Autodesk Inventor part; units mm, degrees
ref_plane "YZ Plane" through (0, 0, 0) normal (1, 0, 0) x (0, 1, 0)
ref_plane "XZ Plane" through (0, 0, 0) normal (0, 1, 0) x (-1, 0, 0)
ref_plane "XY Plane" through (0, 0, 0) normal (0, 0, 1) x (1, 0, 0)
sketch "Sketch1" plane through (0, 0, 0) normal (0, 0, 1) x (1, 0, 0)
  line L0 (-4, 26) -> (-4, -4)
  line L1 (-4, -4) -> (16, -4)
  line L2 (16, -4) -> (16, 0)
  line L3 (16, 0) -> (0, 0)
  line L4 (0, 0) -> (0, 26)
  line L5 (0, 26) -> (-4, 26)
  point P0 (0, 0)
  dimension "d0" = 30
  dimension "d1" = 20
  dimension "d2" = 4
  dimension "d3" = 4
extrude "Extrusion1" add sketch "Sketch1" along normal mid plane 120
sketch "Sketch2" plane through (0, 0, 0) normal (0, 0, 1) x (1, 0, 0)
  line L0 (0, 0) -> (0, 26)
  line L1 (16, -4) -> (16, 0)
  line L2 (0, 26) -> (16, 0)
  line L3 (16, 0) -> (0, 0)
extrude "Extrusion2" add sketch "Sketch2" along normal mid plane 4
fillet "Fillet1" radius 2 8 edges at (0, 0, 31) (0, 0, -31) (0, 13, 2) (8, 0, 2) (0, 13, -2) (8, 0, -2) (-2, 26, 60) (-2, 26, -60)
sketch "Sketch3" plane through (0, 2, 4) normal (1, 0, 0) x (0, 0, -1)
  line L0 (64, -6) -> (-56, -6)
  line L1 (8, 24) -> (0, 24)
  point P0 (4, -2)
  point P1 (-38.5, 12.28)
  point P2 (4, 24)
  dimension "d19" = 18.28
  dimension "d20" = 42.5
hole "Hole1" at (0, 14.28, 42.5) direction (-1, 0, 0) diameter 5.1 depth 4
mirror "Mirror1" about plane through (0, 0, 0) normal (0, 0, 1) of "Hole1"
sketch "Sketch4" plane through (2, 0, 4) normal (0, 1, 0) x (1, 0, 0)
  line L0 (14, 0) -> (14, -56)
  line L1 (14, 8) -> (14, 0)
  point P0 (-2, 4)
  point P1 (4, -28.5)
  point P2 (14, -50)
  point P3 (14, 4)
  dimension "d28" = 10
  dimension "d29" = 32.5
hole "Hole2" at (6, 0, 32.5) direction (0, -1, 0) diameter 3.1 depth 4
mirror "Mirror2" about plane through (0, 0, 0) normal (0, 0, 1) of "Hole2"
sketch "Sketch5" plane through (-4, -4, -60) normal (-1, 0, 0) x (0, 0, 1)
  circle A0 centre (89, 18.28) radius 1.85
  line L0 (144, 18.28) -> (-24, 18.28)
  line L1 (120, 28) -> (120, 0)
  circle A1 centre (29.5, 18.28) radius 1.85
  circle A2 centre (17.5, 18.28) radius 2.55
  point P0 (60, 4)
  dimension "d31" = 3.7
  dimension "d32" = 31
  dimension "d33" = 3.7
  dimension "d34" = 12
extrude "Extrusion3" add sketch "Sketch5" along normal blind 3 contours L0 A0 | A0 L0 | A1 L0 | L0 A1
fillet "Fillet2" radius 1 2 edges at (-7, 14.28, -32.35) (-7, 14.28, 27.15)
properties part number "LV_Bracket_2"
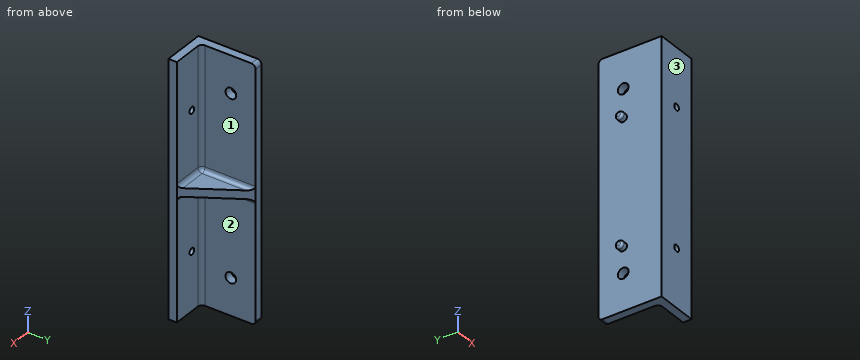
Model file for the job. Use its own axes, mm. Face numbers are marked on the shaded views. A direction names the side the tool comes from. Give positions to 0.01 mm unless a question says otherwise; leave off trailing zeros. Order: outer loops, then holes, each group sorted by start corner. A loop starts at its lowest first (then second) coordinate and runs counter-clockwise, first axis right, second up. Notation, with made-up numbers: M 27,4.5 L 58,4.5 A23 ccw 58,27.5 Z; hole C 70,88 d2. An arc over 180 degrees is marked long. Put each result on its own line as item: value. Start each with the question number.
(1) Pin check, flat tips, straight feed: pin 1 Ø6 at (y, z) = (22, 23.5) entering from +X; pin 2 Ø8 at (y, z) = (8, -5.5) entering from +X; pin 3 Ø3 at (x, y) = (2, 16.5) entering from +Z. Stop position of each tip, or through.
(2) Band-saw the part on C-C on y = 10. Give the cut face in (x, z), then the cut area to 3 significant figures.
(3) Band-saw the part on A-A on z = 42.5. Give the cut face in (x, y), then the cut area to 3 significant figures.
(4) Drill centre lines: L1, parallel to Z at x = 6, y = -3.1; L2, parallel to Z at x = -2.7, y = 14.28; L3, parallel to Z at x = -4.75, y = 14.25. Where is each one in solid material? Low to high. Write a range as [from, to].
(5) Tool access for the marked faces 1, 2 and 3: list every direction of +Z, -Z, +X, -X, +Y, -Y with a clear straight run to the whole face (end or side of a thin tool).
(6) Band-saw the part on B-B on y = 5.5. Give the cut face in (x, z).
Results below:
1. pin 1: stops at x = 0
1. pin 2: stops at x = 12.27
1. pin 3: stops at z = 2.68
2. outline: M -4,-60 L 0,-60 L 0,-4 A2 cw 2,-2 L 9.85,-2 L 9.85,2 L 2,2 A2 cw 0,4 L 0,60 L -4,60 Z
2. area: 521 mm2
3. outline: M -4,-4 L 16,-4 L 16,0 L 2,0 A2 cw 0,2 L 0,11.73 L -4,11.73 Z; M -4,16.83 L 0,16.83 L 0,26 L -4,26 Z
3. area: 164 mm2
4. L1: z = [-60, -34.05], [-30.95, 30.95], [34.05, 60]
4. L2: z = [-60, -45.05], [-39.95, 39.95], [45.05, 60]
4. L3: z = [-32.35, -28.65], [27.15, 30.85]
5. face 1: +Z, +X, +Y
5. face 2: -Z, +X, +Y
5. face 3: +Z, -Z, +X, -X, -Y
6. outline: M -4,-60 L 0,-60 L 0,-4 A2 cw 2,-2 L 12.62,-2 L 12.62,2 L 2,2 A2 cw 0,4 L 0,60 L -4,60 Z
